```python
from build123d import *

# Parameters (mm, degrees)
SALIENTE_EXTRUIR1_DEPTH = 11
CORTAR_EXTRUIR1_DEPTH   = 61
CROQUIS3_W              = 6.95445115
CROQUIS3_H              = 10
CORTAR_EXTRUIR2_DEPTH   = 61
CROQUIS4_R              = 1.2
CORTAR_EXTRUIR3_DEPTH   = 61
CROQUIS5_R              = 1.5
SALIENTE_EXTRUIR2_DEPTH = 1.5
REDONDEO2_SIZE          = 1
REDONDEO6_SIZE          = 1
CROQUIS6_W              = 1
CROQUIS6_H              = 11
CORTAR_EXTRUIR4_DEPTH   = 2
CROQUIS7_W              = 1
CROQUIS7_H              = 11
CORTAR_EXTRUIR5_DEPTH   = 2


with BuildPart() as part:
    # Croquis1 → Saliente-Extruir1 (new body)
    with BuildSketch(Plane.XY):
        Polygon((-5, 7), (5, 7), (5, 9), (5.755229402, 9), (27, -6), (27, -9), (5, -9), (5, -7), (-5, -7), (-5, -5), (0, -5), (0, 5), (-5, 5), align=None)
    extrude(amount=SALIENTE_EXTRUIR1_DEPTH)

    # Croquis2 → Cortar-Extruir1 (cut)
    with BuildSketch(Plane.XZ.offset(7)):
        with BuildLine():
            ThreePointArc((-5, 5.5), (-3.389087297, 9.389087297), (0.5, 11))
            Line((0.5, 11), (-5, 11))
            Line((-5, 11), (-5, 5.5))
        make_face()
        with BuildLine():
            ThreePointArc((0.5, 0), (-3.389087297, 1.610912703), (-5, 5.5))
            Line((-5, 5.5), (-5, 0))
            Line((-5, 0), (0.5, 0))
        make_face()
    extrude(amount=-CORTAR_EXTRUIR1_DEPTH, mode=Mode.SUBTRACT)

    # Croquis3 → Cortar-Extruir2 (cut)
    with BuildSketch(Plane.ZY):
        with Locations((5.5, 0)):
            Rectangle(CROQUIS3_W, CROQUIS3_H)
    extrude(amount=-CORTAR_EXTRUIR2_DEPTH, mode=Mode.SUBTRACT)

    # Croquis4 → Cortar-Extruir3 (cut)
    with BuildSketch(Plane(origin=(0, -5, 0), x_dir=(1, 0, 0), z_dir=(0, 1, 0))):
        with Locations(Location((22.58368196, -5.5, 0), (0, 0, 270))):
            Circle(CROQUIS4_R)
        with Locations(Location((16.58368196, -5.5, 0), (0, 0, 270))):
            Circle(CROQUIS4_R)
    extrude(amount=-CORTAR_EXTRUIR3_DEPTH, mode=Mode.SUBTRACT)

    # Croquis5 → Saliente-Extruir2 (add)
    with BuildSketch(Plane(origin=(0, 7, 0), x_dir=(1, 0, 0), z_dir=(0, 1, 0))):
        with Locations((0.5, -5.5)):
            Circle(CROQUIS5_R)
    saliente_extruir2 = extrude(amount=SALIENTE_EXTRUIR2_DEPTH)

    # Simetría4: Saliente-Extruir2 across plane
    add(saliente_extruir2.mirror(Plane.ZX))

    # Redondeo2
    # a fillet whose section is not a circle: 1 mm, written as the material it takes off along each edge
    with BuildSketch(Plane(origin=(0.5, 8.5, 5.5), x_dir=(1, 0, 0), z_dir=(0, 0, 1))) as redondeo2_piece_1:
        with BuildLine():
            Bezier((1.5, -REDONDEO2_SIZE), (1.5, 0), (1.5 - REDONDEO2_SIZE, 0), weights=[1, 0.141421356, 1])
            Line((1.5 - REDONDEO2_SIZE, 0), (1.5, 0))
            Line((1.5, 0), (1.5, -REDONDEO2_SIZE))
        make_face()
    revolve(axis=Axis((0.5, 8.5, 5.5), (0, 1, 0)), mode=Mode.SUBTRACT)

    # Redondeo6
    # a fillet whose section is not a circle: 1 mm, written as the material it takes off along each edge
    with BuildSketch(Plane(origin=(0.5, -8.5, 5.5), x_dir=(1, 0, 0), z_dir=(0, 0, 1))) as redondeo6_piece_1:
        with BuildLine():
            Bezier((1.5, REDONDEO6_SIZE), (1.5, 0), (1.5 - REDONDEO6_SIZE, 0), weights=[1, 0.141421356, 1])
            Line((1.5 - REDONDEO6_SIZE, 0), (1.5, 0))
            Line((1.5, 0), (1.5, REDONDEO6_SIZE))
        make_face()
    revolve(axis=Axis((0.5, -8.5, 5.5), (0, 1, 0)), mode=Mode.SUBTRACT)

    # Croquis6 → Cortar-Extruir4 (cut)
    with BuildSketch(Plane(origin=(0, 9, 0), x_dir=(1, 0, 0), z_dir=(0, 1, 0))):
        with Locations((5.5, -5.5)):
            Rectangle(CROQUIS6_W, CROQUIS6_H)
    extrude(amount=-CORTAR_EXTRUIR4_DEPTH, mode=Mode.SUBTRACT)

    # Croquis7 → Cortar-Extruir5 (cut)
    with BuildSketch(Plane.XZ.offset(9)):
        with Locations((5.5, 5.5)):
            Rectangle(CROQUIS7_W, CROQUIS7_H)
    extrude(amount=-CORTAR_EXTRUIR5_DEPTH, mode=Mode.SUBTRACT)


solid = part.part
```
CAD build for the part. Positions are in the model's coordinates, mm. A direction names the side the tool comes from. Round coordinates to 2 decimals unless told otherwise and drop trailing zeros. Order: outer loops, then holes, each group sorted by start corner. A loop starts at its lowest first (then second) coordinate and runs counter-clockwise, first axis right, second up. Notation, with made-up numbers: (46, -38.75) -> (76, -38.75) arc R19 cw to (76, -7.75) -> close; hole circle Ø10 at (-31.75, 45). An arc over 180 degrees is marked (long way). Write item = value, one per line.
(1) Drill centre lines: L1, parallel to X at y = -6.95, z = 5.5; L2, parallel to Y at x = 2, z = 3; L3, parallel to X at y = -7.4, z = 5.5. Where is each one in solid material? Low to high.
Answers follow:
L1 = -5 to 15.38, 17.78 to 21.38, 23.78 to 27
L2 = -7 to -5, 5 to 7
L3 = -1 to 2, 6 to 15.38, 17.78 to 21.38, 23.78 to 27
(2) Pull direction Y, two halves, no side cores. Call faces 5 (the flat face through (3, 5, 5)), 6 (the flat face through (2, -7, 7)), 7 (the flat face through (16.35, 1.52, 1.76)): +Y half, -Y half, draft (parallel to the pull), parting line (faces both ways), or undercut.
Answers follow:
face_5 = undercut
face_6 = -Y half
face_7 = +Y half
(3) Cut at B-B (y = 1.5). Write the cut outline in (x, z), plus the area to 3 significant figures.
Answers follow:
outline = (0, 0.02) arc R5.5 ccw to (0.5, 0) -> (16.38, 0) -> (16.38, 2.02) -> (0, 2.02) -> close; (0, 8.98) -> (16.38, 8.98) -> (16.38, 11) -> (0.5, 11) arc R5.5 ccw to (0, 10.98) -> close
area = 66.2 mm²
(4) 3-axis set-ups, long thin cutter, end or side, ignore diameter. For faces 1 (the flat face through (10, -1, 8.977)), 2 (the flat face through (0, 0, 1)), 3 (the flat face through (7, -5, 5)), 4 (the flat face through (0.5, -8.5, 5.5)): which of +Z, -Z, +X, -X, +Y, -Y reach the whole face in a straight line?
Answers follow:
face_1 = +X, -X
face_2 = +Z, -Z, -X
face_3 = -X
face_4 = +Z, -Z, -X, -Y
(5) Cut at C-C (x = 9). Write the cut outline in (y, z).
Answers follow:
outline = (-9, 0) -> (6.71, 0) -> (6.71, 11) -> (-9, 11) -> close; hole (-5, 2.02) -> (5, 2.02) -> (5, 8.98) -> (-5, 8.98) -> close
(6) Flat gauge pins, fed straight in: P1, Ø1.5, axis at x = 6.5, z = 8, coming from the +Y side; P2, Ø0.6, axis at y = -1.5, z = 1, coming from the -X side; P3, Ø0.9, axis at y = 8, z = 6, coming from the -X side; P4, Ø8, axis at x = 17.5, y = -1, coming from the -Z side. Where does each tip first touch, or does it go through?
Answers follow:
P1 = 8.83
P2 = 0
P3 = -0.93
P4 = 0
(7) Cut at D-D (x = 13). Write the cut outline in (y, z), plus the area to 3 significant figures.
Answers follow:
outline = (-9, 0) -> (3.88, 0) -> (3.88, 2.02) -> (-5, 2.02) -> (-5, 8.98) -> (3.88, 8.98) -> (3.88, 11) -> (-9, 11) -> close
area = 79.9 mm²
(8) Cut at A-A (z = 2.5). Write the cut outline in (x, y), plus the area to 3 significant figures.
Answers follow:
outline = (-4.11, -7) -> (6, -7) -> (6, -9) -> (27, -9) -> (27, -6) -> (25.58, -5) -> (-4.11, -5) -> close; (-4.11, 5) -> (11.42, 5) -> (6, 8.83) -> (6, 7) -> (-4.11, 7) -> close
area = 134 mm²
